from build123d import *

# Parameters (mm, degrees)
BOSS_EXTRUDE1_DEPTH                             = 3.175
CSK_FOR_M3_FLAT_HEAD_MACHINE_SCREW1_D           = 3.4
CSK_FOR_M3_FLAT_HEAD_MACHINE_SCREW1_CSINK_D     = 6.3
CSK_FOR_M3_FLAT_HEAD_MACHINE_SCREW1_CSINK_ANGLE = 90


with BuildPart() as part:
    # Sketch1 → Boss-Extrude1 (new body)
    with BuildSketch(Plane(origin=(0, 0, 0), x_dir=(0, 0, -1), z_dir=(1, 0, 0))):
        with BuildLine():
            Line((-100, 0), (100, 0))
            Line((100, 0), (100, 57.35))
            ThreePointArc((100, 57.35), (99.121320344, 59.471320344), (97, 60.35))
            Line((97, 60.35), (-97, 60.35))
            ThreePointArc((-97, 60.35), (-99.121320344, 59.471320344), (-100, 57.35))
            Line((-100, 57.35), (-100, 0))
        make_face()
    extrude(amount=BOSS_EXTRUDE1_DEPTH)

    # CSK for M3 Flat Head Machine Screw1 (through all)
    with Locations(Plane(origin=(3.175, 0, 0), x_dir=(0, 0, -1), z_dir=(1, 0, 0))):
        with Locations((-95, 8.175), (-95, 55.35)):
            csk_for_m3_flat_head_machine_screw1 = CounterSinkHole(CSK_FOR_M3_FLAT_HEAD_MACHINE_SCREW1_D / 2, CSK_FOR_M3_FLAT_HEAD_MACHINE_SCREW1_CSINK_D / 2, counter_sink_angle=CSK_FOR_M3_FLAT_HEAD_MACHINE_SCREW1_CSINK_ANGLE)

    # Mirror1: CSK for M3 Flat Head Machine Screw1 across plane
    add(csk_for_m3_flat_head_machine_screw1.mirror(Plane.XY), mode=Mode.SUBTRACT)


solid = part.part
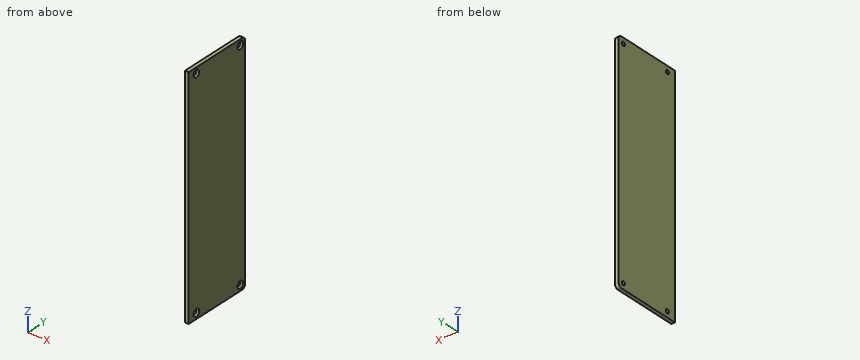
The model under review builds one solid part; all positions refer to its coordinate system, in mm. Give positions to 0.01 mm unless a question says otherwise; leave off trailing zeros. Order: outer loops, then holes, each group sorted by start corner. A loop starts at its lowest first (then second) coordinate and runs counter-clockwise, first axis right, second up. Notation, with made-up numbers: M 70,-24.75 L 124,-24.75 A18 cw 124,-14.75 Z; hole C 33.5,30 d6. An arc over 180 degrees is marked long. Answer in a Markdown table with one row per item. Add a question column.
1. Add section A-A on y = 55.35. State the section outline as (x, z) points (3 decimals).
2. For pin 1 Ø4.5 at (y, z) = (55.35, 95) entering from +X (3 decimals); pin 2 Ø2 at (y, z) = (55.35, -95) entering from -X, all flat-tipped, find the tip position at first contact; note any pin that passes through.
3. To check wall thickness, follow line 1 along Y through (x, z) = (0.75, -95) (3 decimals); line 2 along Z through (x, y) = (0.95, 55.35). State the ranges of each line that lie inside material, in increasing order.
4. Add section B-B on z = 95. State the section outline as (x, y) points (3 decimals).
The answers:
| question | item | result |
|---|---|---|
| 1 | outline | M 0,-100 L 3.175,-100 L 3.175,-98.15 L 1.725,-96.7 L 0,-96.7 Z; M 0,-93.3 L 1.725,-93.3 L 3.175,-91.85 L 3.175,91.85 L 1.725,93.3 L 0,93.3 Z; M 0,96.7 L 1.725,96.7 L 3.175,98.15 L 3.175,100 L 0,100 Z |
| 2 | pin 1 | x = 2.275 |
| 2 | pin 2 | through |
| 3 | line 1 | 0 to 6.475, 9.875 to 53.65, 57.05 to 60.35 |
| 3 | line 2 | -100 to -96.7, -93.3 to 93.3, 96.7 to 100 |
| 4 | outline | M 0,0 L 3.175,0 L 3.175,5.025 L 1.725,6.475 L 0,6.475 Z; M 0,9.875 L 1.725,9.875 L 3.175,11.325 L 3.175,52.2 L 1.725,53.65 L 0,53.65 Z; M 0,57.05 L 1.725,57.05 L 3.175,58.5 L 3.175,60.35 L 0,60.35 Z |
